Could you check a few things on this drawing? It's one solid part, dimensions in mm from its lowest x, y, z. A direction names the side the tool comes from. Coordinates: 2 decimals unless noted, no trailing zeros. Write each loop counter-clockwise with the first axis right and the second up, starting at its lowest first coordinate (ties: lowest second). Pieces come first, ordered by that corner, then holes.
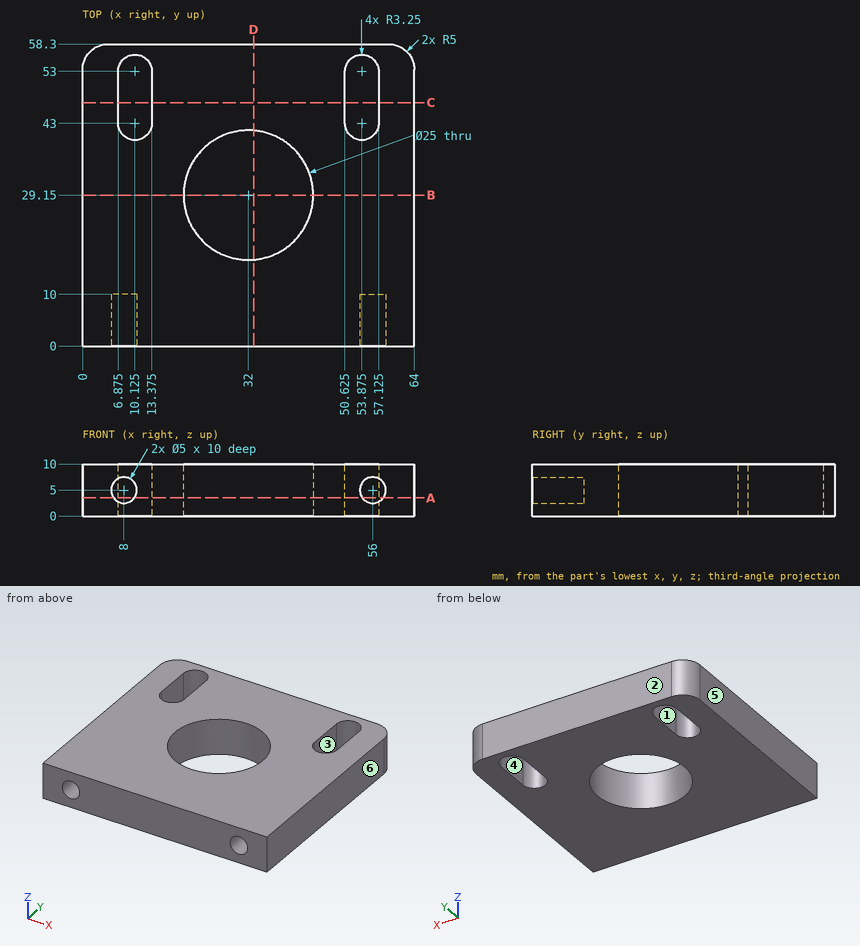
1) Imagine slicing it at C-C on y = 47. Please give me the cut outline in (x, z) (3 decimals), then the cut area to 3 significant figures.
Values follow:
outline: (0, 0) - (6.875, 0) - (6.875, 10) - (0, 10) - close; (13.375, 0) - (50.625, 0) - (50.625, 10) - (13.375, 10) - close; (57.125, 0) - (64, 0) - (64, 10) - (57.125, 10) - close
area: 510 mm2
2) On a 3-axis mill with a long thin cutter (end or side, diameter ignored), from which of +Z, -Z, +X, -X, +Y, -Y can I reach the whole of each face in a straight line? I mean the marked faces 1 and 2. Say none if no direction works.
Values follow:
face 1: +Z, -Z
face 2: +Z, -Z, +X, -X, +Y
3) I need wall thicknesses on probe 1 along X at (y, z) = (8.5, 4.75); probe 2 along X at (y, z) = (46.5, 1.5) (3 decimals); probe 3 along Z at (x, y) = (56, 6.5). Which ranges of each line are inside material? Lowest first, please.
Values follow:
probe 1: x = 0 to 5.51, 10.49 to 53.51, 58.49 to 64
probe 2: x = 0 to 6.875, 13.375 to 50.625, 57.125 to 64
probe 3: z = 0 to 2.5, 7.5 to 10
4) Imagine slicing it at B-B on y = 29.15. Please give me the cut outline in (x, z), then the cut area to 3 significant figures.
Values follow:
outline: (0, 0) - (19.5, 0) - (19.5, 10) - (0, 10) - close; (44.5, 0) - (64, 0) - (64, 10) - (44.5, 10) - close
area: 390 mm2
5) Will this pin go through, and if not, where does the flat tip stop? pin 1 (3 mm diameter, centred on x = 8, z = 5, fed in from -Y).
Values follow:
pin 1: stops at y = 10
6) We'd pull the mould along X, two halves only. Please class the marked faces 3, 4, 5 and 6: pulls with the +X half, pulls with the -X half, needs draft (parallel to the pull), parting line crosses it, or undercut.
Values follow:
face 3: undercut
face 4: undercut
face 5: pulls with the -X half
face 6: pulls with the +X half
7) Imagine slicing it at A-A on z = 3.5. Please give me the cut outline in (x, y) (3 decimals), then the cut area to 3 significant figures.
Values follow:
outline: (0, 0) - (6, 0) - (6, 10) - (10, 10) - (10, 0) - (54, 0) - (54, 10) - (58, 10) - (58, 0) - (64, 0) - (64, 53.3) arc R5 ccw to (59, 58.3) - (5, 58.3) arc R5 ccw to (0, 53.3) - close; hole (6.875, 43) arc R3.25 ccw to (13.375, 43) - (13.375, 53) arc R3.25 ccw to (6.875, 53) - close; hole circle Ø25 at (32, 29.15); hole (50.625, 43) arc R3.25 ccw to (57.125, 43) - (57.125, 53) arc R3.25 ccw to (50.625, 53) - close
area: 2,950 mm2
8) Imagine slicing it at D-D on x = 33. Please give me the cut outline in (y, z), then the cut area to 3 significant figures.
Values follow:
outline: (0, 0) - (16.69, 0) - (16.69, 10) - (0, 10) - close; (41.61, 0) - (58.3, 0) - (58.3, 10) - (41.61, 10) - close
area: 334 mm2
